Verification items for this drawing (mm, ordinates from the low corner). A direction names the side the tool comes from. Give positions to 0.01 mm unless a question says otherwise; leave off trailing zeros. Order: outer loops, then holes, each group sorted by start corner. A loop starts at its lowest first (then second) coordinate and runs counter-clockwise, first axis right, second up.
(1) Sectioned sample at A-A on y = 21. Record the cut outline in (x, z).
(2) Sectioned sample at B-B on x = 29.5. Record the cut outline in (y, z), plus the area to 3 significant figures.
(3) Sectioned sample at D-D on y = 27.5. Record the cut outline in (x, z).
(4) Access from +Z, -Z, +X, -X, +Y, -Y to the whole of each face (thin tool, end or side, straight path). Record for the marked faces 1 and 2.
(5) Gauge pin test, flat ends, axial feed: pin 1 (10 mm diameter, centred on x = 36.5, y = 29, fed in from -Z); pin 2 (3 mm diameter, centred on x = 21.5, z = 11, fed in from -Y). Record the tip position at first contact, or that the pin passes through.
(6) Scan lines: L1, parallel to Z at x = 19, y = 2; L2, parallel to Y at x = 21, z = 13; L3, parallel to Z at x = 14.5, y = 12. Record each from-to range of solid material in increasing order.
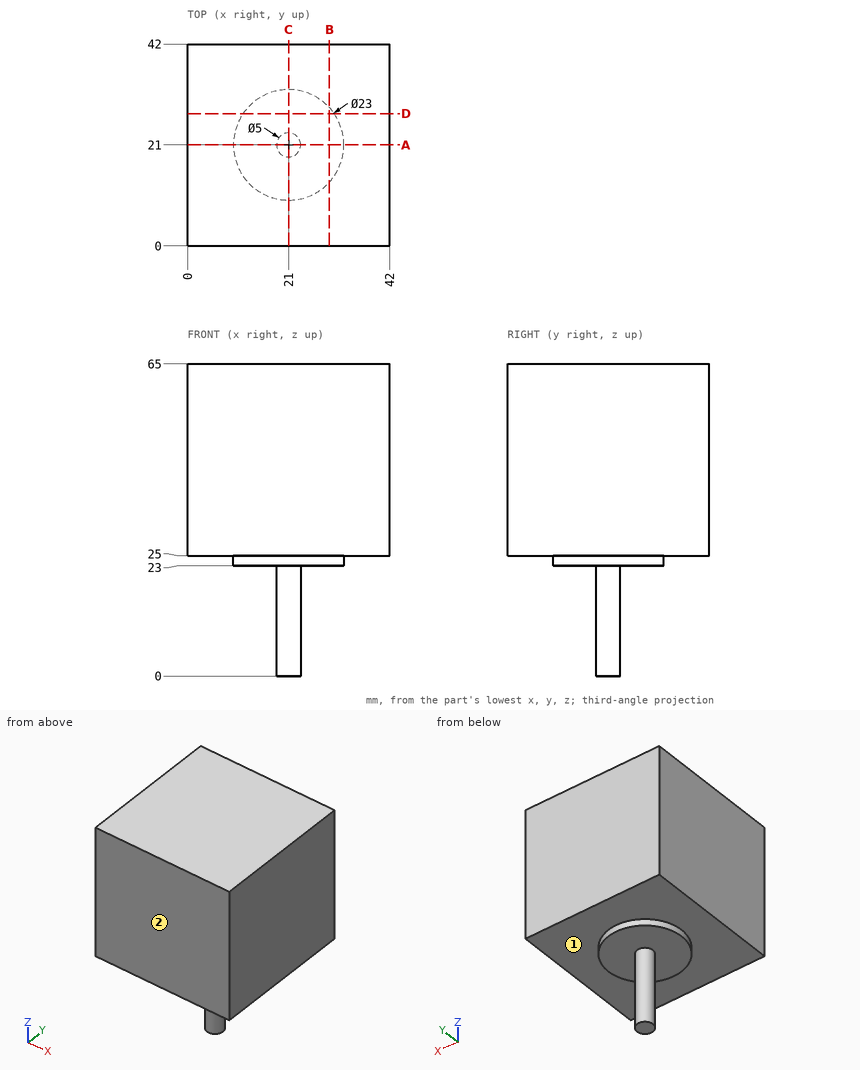
Ans:
1. outline: (0, 25) - (9.5, 25) - (9.5, 23) - (18.5, 23) - (18.5, 0) - (23.5, 0) - (23.5, 23) - (32.5, 23) - (32.5, 25) - (42, 25) - (42, 65) - (0, 65) - close
2. outline: (0, 25) - (13.25, 25) - (13.25, 23) - (28.75, 23) - (28.75, 25) - (42, 25) - (42, 65) - (0, 65) - close
2. area: 1,710 mm2
3. outline: (0, 25) - (11.51, 25) - (11.51, 23) - (30.49, 23) - (30.49, 25) - (42, 25) - (42, 65) - (0, 65) - close
4. face 1: -Z
4. face 2: +Z, -Z, +X, -X, -Y
5. pin 1: stops at z = 25
5. pin 2: stops at y = 18.5
6. L1: z = 25 to 65
6. L2: y = 18.5 to 23.5
6. L3: z = 23 to 65
